```python
from build123d import *

# Parameters (mm, degrees)
BOSS_EXTRUDE1_DEPTH = 82
CUT_EXTRUDE1_DEPTH  = 105
SKETCH7_W           = 23
SKETCH7_H           = 43
CUT_EXTRUDE3_DEPTH  = 28
CUT_EXTRUDE4_DEPTH  = 32
CUT_EXTRUDE5_DEPTH  = 32
CUT_EXTRUDE6_DEPTH  = 32


with BuildPart() as part:
    # Sketch1 → Boss-Extrude1 (new body)
    with BuildSketch(Plane(origin=(0, 0, 0), x_dir=(1, 0, 0), z_dir=(0, 1, 0))):
        with BuildLine():
            Line((-21.9286378, 20.529965557), (30.819410356, 20.529965557))
            Line((30.819410356, 20.529965557), (30.819410356, 8.269460429))
            ThreePointArc((30.819410356, 8.269460429), (29.737157279, 6.984989328), (28.898083391, 5.52996605))
            Line((28.898083391, 5.52996605), (24.81959218, 5.52996605))
            Line((24.81959218, 5.52996605), (14.820019426, -17.47003395))
            Line((14.820019426, -17.47003395), (3.320446672, -17.47003395))
            ThreePointArc((3.320446672, -17.47003395), (-2.977277813, -22.983126936), (-11.218310652, -24.446310348))
            ThreePointArc((-11.218310652, -24.446310348), (-19.829053504, -21.990642561), (-25.924914656, -15.432009048))
            Line((-25.924914656, -15.432009048), (-26.328479109, -14.47003395))
            Line((-26.328479109, -14.47003395), (-25.288623152, -0.544399566))
            Line((-25.288623152, -0.544399566), (-24.844287214, 3.45451706))
            Line((-24.844287214, 3.45451706), (-24.102893172, 7.451406174))
            Line((-24.102893172, 7.451406174), (-23.328601179, 10.529965096))
            Line((-23.328601179, 10.529965096), (-22.928576765, 16.529967242))
            Line((-22.928576765, 16.529967242), (-22.928576765, 18.529964858))
            Line((-22.928576765, 18.529964858), (-21.9286378, 20.529965557))
        make_face()
    extrude(amount=BOSS_EXTRUDE1_DEPTH)

    # Sketch2 → Cut-Extrude1 (cut)
    with BuildSketch(Plane.XZ):
        Polygon((-18.173439963, -16.784486826), (-18.173439963, 15.715513413), (-3.173989279, 15.715513413), (-3.173989279, 13.315508549), (9.57552244, 13.315508549), (9.57552244, -14.3844853), (-3.173989279, -14.3844853), (-3.173989279, -16.784486826), align=None)
    extrude(amount=-CUT_EXTRUDE1_DEPTH, mode=Mode.SUBTRACT)

    # Sketch7 → Cut-Extrude3 (cut)
    with BuildSketch(Plane(origin=(40, 0, 0), x_dir=(0, 0, -1), z_dir=(1, 0, 0))):
        with Locations((-5.97003395, 28.5)):
            Rectangle(SKETCH7_W, SKETCH7_H)
    extrude(amount=-CUT_EXTRUDE3_DEPTH, mode=Mode.SUBTRACT)

    # Sketch9 → Cut-Extrude4 (cut)
    with BuildSketch(Plane(origin=(0, 82, 0), x_dir=(1, 0, 0), z_dir=(0, 1, 0))):
        Polygon((14.820019426, -17.47003395), (24.81959218, 5.52996605), (15.399238031, 5.52996605), align=None)
    extrude(amount=-CUT_EXTRUDE4_DEPTH, mode=Mode.SUBTRACT)

    # Sketch10 → Cut-Extrude5 (cut)
    with BuildSketch(Plane(origin=(0, 82, 0), x_dir=(1, 0, 0), z_dir=(0, 1, 0))):
        Polygon((3.320446672, -17.47003395), (3.20076658, -13.315508549), (9.57552244, -13.315508549), (9.57552244, 14.3844853), (9.57552244, 18.3844853), (27.57552244, 18.3844853), (27.57552244, 9.3844853), (27.57552244, 5.52996605), (15.399238031, 5.52996605), (14.820019426, -17.47003395), align=None)
    extrude(amount=-CUT_EXTRUDE5_DEPTH, mode=Mode.SUBTRACT)

    # Sketch12 → Cut-Extrude6 (cut)
    with BuildSketch(Plane(origin=(0, 82, 0), x_dir=(1, 0, 0), z_dir=(0, 1, 0))):
        Polygon((9.57552244, 14.3844853), (-3.173989279, 14.3844853), (-3.173989279, 16.784486826), (-18.173439963, 16.784486826), (-18.173439963, 18.3844853), (9.57552244, 18.3844853), align=None)
    extrude(amount=-CUT_EXTRUDE6_DEPTH, mode=Mode.SUBTRACT)


solid = part.part
```
Source: CAD feature listing. Evaluate the final solid. Frame: model axes, mm. A direction names the side the tool comes from. Give positions to 0.01 mm unless a question says otherwise; leave off trailing zeros. Write each loop counter-clockwise with the first axis right and the second up, starting at its lowest first coordinate (ties: lowest second). Pieces come first, ordered by that corner, then holes. Notation, with made-up numbers: (-21.75, 40) - (-11.75, 40) arc R15 ccw to (-11.75, 50) - close; hole circle Ø7 at (-15.5, 25). An arc over 180 degrees is marked (long way). One line per item, written item: value. Start each with the question number.
Q1. Set-up query: faces 1 (the face through (8, 25, 17.47)), 2 (the face through (-11, 40, 15.716)), 3 (the face through (4, 66, -18.384)). Return all of +Z, -Z, +X, -X, +Y, -Y with unobstructed straight access to the full face (end or side cutting, diameter ignored); none if empty.
Q2. First-contact query: pin 1 Ø11 at (x, z) = (7.5, 4) entering from +Y; pin 2 Ø6.5 at (x, y) = (2.5, 26.5) entering from +Z; pin 3 Ø12.5 at (x, y) = (9.5, 15.5) entering from +Z; pin 4 Ø4 at (x, z) = (6.5, -6.5) entering from +Y. Flat tips, straight axial feed; report the tip coordinate or a pass-through.
Q3. Section query A-A, the plane x = 6.5. Return the cut outline in (y, z), then the cut area to 3 significant figures.
Q4. Section query D-D, the plane y = 11.5. Return the cut outline in (x, z).
Q5. Section query C-C, the plane z = 4. Return the cut outline in (x, y), then the cut area to 3 significant figures.
Q6. Section query B-B, the plane y = 66. Return the cut outline in (x, z), then the cut area to 3 significant figures.
Q7. Material intervals for probe 1 along X at (y, z) = (60.5, -16.5); probe 2 along Z at (x, y) = (5, 48.5); probe 3 along Z at (x, y) = (5.5, 52), sorted ascending. Write a range as from..to.
Q8. Draft query along Z for faces 4 (the face through (30.819, 40, -14)), 5 (the face through (-25.07, 40.43, -1.43)), 6 (the face through (3, 25, -14.384)). Return one class per face: +Z half, -Z half, draft (parallel to the pull), parting line (faces both ways), or undercut.
Answer:
1. face 1: +Z, +X, +Y, -Y
1. face 2: +Y, -Y
1. face 3: +Y
2. pin 1: stops at y = 50
2. pin 2: stops at z = 21.68
2. pin 3: stops at z = 17.58
2. pin 4: passes through
3. outline: (0, -20.53) - (82, -20.53) - (82, -18.38) - (50, -18.38) - (50, -14.38) - (0, -14.38) - close; (0, 13.32) - (50, 13.32) - (50, 17.47) - (0, 17.47) - close
3. area: 584 mm2
4. outline: (-26.33, 14.47) - (-25.29, 0.54) - (-24.84, -3.45) - (-24.1, -7.45) - (-23.33, -10.53) - (-22.93, -16.53) - (-22.93, -18.53) - (-21.93, -20.53) - (30.82, -20.53) - (30.82, -8.27) arc R9.5 cw to (28.9, -5.53) - (12, -5.53) - (12, 17.47) - (3.32, 17.47) arc R15.6 ccw to (-11.22, 24.45) arc R16.66 ccw to (-25.92, 15.43) - close; hole (-18.17, -16.78) - (-3.17, -16.78) - (-3.17, -14.38) - (9.58, -14.38) - (9.58, 13.32) - (-3.17, 13.32) - (-3.17, 15.72) - (-18.17, 15.72) - close
5. outline: (-25.55, 0) - (-18.17, 0) - (-18.17, 82) - (-25.55, 82) - close; (9.58, 0) - (20.68, 0) - (20.68, 7) - (12, 7) - (12, 50) - (9.58, 50) - close
5. area: 787 mm2
6. outline: (-26.33, 14.47) - (-25.29, 0.54) - (-24.84, -3.45) - (-24.1, -7.45) - (-23.33, -10.53) - (-22.93, -16.53) - (-22.93, -18.53) - (-21.93, -20.53) - (30.82, -20.53) - (30.82, -8.27) arc R9.5 cw to (28.9, -5.53) - (27.58, -5.53) - (27.58, -18.38) - (-18.17, -18.38) - (-18.17, 15.72) - (-3.17, 15.72) - (-3.17, 13.32) - (3.2, 13.32) - (3.32, 17.47) arc R15.6 ccw to (-11.22, 24.45) arc R16.66 ccw to (-25.92, 15.43) - close
6. area: 584 mm2
7. probe 1: x = -22.93..-18.17, 27.58..30.82
7. probe 2: z = -20.53..-14.38, 13.32..17.47
7. probe 3: z = -20.53..-18.38
8. face 4: draft
8. face 5: -Z half
8. face 6: undercut
